The listing builds one solid part. Answer for the finished solid, in the listing's coordinates (mm). A direction names the side the tool comes from. Coordinates: 2 decimals unless noted, no trailing zeros. Order: outer loops, then holes, each group sorted by start corner. A loop starts at its lowest first (then second) coordinate and runs counter-clockwise, first axis right, second up.
from build123d import *

# Parameters (mm, degrees)
F2_SIZE = 20


with BuildPart() as f1:
    # F0 (on Front) → F1 (revolve)
    with BuildSketch(Plane.XZ):
        with BuildLine():
            Line((0, 350.3882980986), (0, -350))
            Line((0, -350), (370.6526133659, -199.6117019014))
            Line((370.6526133659, -199.6117019014), (370.6526133659, -49.6117019014))
            Line((370.6526133659, -49.6117019014), (150.6526133659, -49.6117019014))
            ThreePointArc((150.6526133659, -49.6117019014), (94.084070871, -26.1802443963), (70.6526133659, 30.3882980986))
            Line((70.6526133659, 30.3882980986), (70.6526133659, 350.3882980986))
            Line((70.6526133659, 350.3882980986), (0, 350.3882980986))
        make_face()
    revolve(axis=Axis((0, 0, 0.1941490493), (0, 0, -1)))

    # F2
    f2_edges = [f1.edges().sort_by_distance(p)[0] for p in [
        (-70.652613, 0, 350.388298),
    ]]
    chamfer(f2_edges, length=F2_SIZE)


solid = f1.part
1) Each of these flat-tipped pins is pushed along its axis until it touches: P1, Ø4, axis at y = 237.5, z = -173.5, coming from the -X side; P2, Ø2, axis at x = 67.5, y = -97.5, coming from the +Z side; P3, Ø1.5, axis at x = 86.5, z = -113.5, coming from the +Y side. Where does it stop, or does it pass through?
2) Section A-A (z = -156.5) is taken. Give the vertices of the cut face in (x, y), then the cut area to 3 significant figures.
3) Consider L1, parallel to Y at x = -49.5, z = 230.5; L2, parallel to Y at x = 13, z = 166.5; L3, parallel to X at y = 32, z = 203. Determine where each line is inside the solid, lowest interval first.
4) Section B-B (z = 0) is taken. Give the vertices of the cut face in (x, y), then the cut area to 3 significant figures.
5) A tool of negligible diameter and unlimited length cuts with its end or side. For faces 1 (the face through (-1, -1, 350.388)), 2 (the face through (67.39, -21.22, 182.49)), from which of +Z, -Z, +X, -X, +Y, -Y can it reach the whole face along a straight path? Write none if from no direction.
Filled sheet:
1. P1: stops at x = -286.22
1. P2: stops at z = -42.46
1. P3: stops at y = 360.6
2. outline: circle Ø741.31 at (0, 0)
2. area: 432,000 mm2
3. L1: y = -50.41 to 50.41
3. L2: y = -69.45 to 69.45
3. L3: x = -62.99 to 62.99
4. outline: circle Ø153.3 at (0, 0)
4. area: 18,500 mm2
5. face 1: +Z, +X, -X, +Y, -Y
5. face 2: +Z
